Input: part model. Units: mm. Frame: model coordinates. A direction names the side the tool comes from. Give positions to 0.01 mm unless a question says otherwise; leave off trailing zeros. Write each loop counter-clockwise with the first axis right and the second up, starting at its lowest first coordinate (ties: lowest second). Pieces come first, ordered by that corner, then holes. Notation, with made-up numbers: (17, 85) -> (28, 85) arc R11 ccw to (28, 92) -> close; hole circle Ø8 at (47, 79). An arc over 180 degrees is marked (long way). Return JSON: item names as keys, results as strings. Group by question number.
Item 1: Section B-B, the plane z = 22. Return loops of the section in (x, y).
Item 2: Pin query (flat end, axial travel): P1, Ø6.5, axis at x = 10.5, y = -16, coming from the +Z side (3 decimals); P2, Ø1, axis at x = 12, y = -6.5, coming from the +Z side; P3, Ø5.5, axis at x = -20.32, y = -20.32, coming from the +Z side; P4, Ø6.5, axis at x = -20.32, y = 20.32, coming from the -Z side. Return the tip coordinate at first contact, or that it passes through.
Item 3: Section C-C, the plane x = 20.32. Return loops of the section in (y, z) (3 decimals), then the cut area to 3 significant figures.
Item 4: Line query: line 1 (Y direction, x = 20.32, z = 1); line 2 (Z direction, x = 13, y = -16.5) (3 decimals). Output: solid intervals per line, ascending. Write a range as [from, to].
Item 5: Section A-A, the plane y = 20.32. Return loops of the section in (x, z) (3 decimals), then the cut area to 3 significant figures.
Item 6: Set-up query: faces 5 (the face through (-25.4, 0, 2)), 6 (the face through (0, -19, 3.175)), 7 (the face through (0, 19, 3.175)). Return all of +Z, -Z, +X, -X, +Y, -Y with unobstructed straight access to the full face (end or side cutting, diameter ignored); none if empty.
Item 7: Section D-D, the plane y = 10.5. Return loops of the section in (x, z) (3 decimals).
Item 8: Mould query, pull axis X, two halves, no side actions, for faces 1 (the face through (17.879, -0.178, 13.234)), 2 (the face through (-19.228, -22.033, 1.19)), 3 (the face through (0, -12.7, 7)), 4 (the face through (18.82, 18.95, 1.19)). Classes: released by +X, released by -X, zero draft, split by the parting line, or undercut.
from build123d import *

# Parameters (mm, degrees)
F0_W        = 50.8
F0_H        = 50.8
F1_DEPTH    = 3.175
F3_DEPTH    = 12.7
F4_T1_DEPTH = 29.6642315955
F5_R        = 2.032
F6_DEPTH    = 25.4
F7_SIZE     = 0.762


# Not quite as in the source:
# - a fillet or chamfer that OpenCascade refuses, or shapes differently, is made with other operations: its cross-section is extruded or revolved along the edge and cut away or added


with BuildPart() as f1:
    # F0 (on Top) → F1 (new body)
    with BuildSketch(Plane.XY):
        Rectangle(F0_W, F0_H)
    extrude(amount=F1_DEPTH)

    # F2 (on Front) → F3 (join, symmetric)
    with BuildSketch(Plane.XZ):
        with BuildLine():
            ThreePointArc((9.6386223082, 24.257), (0, 9.017), (-9.6386223082, 24.257))
            Line((-9.6386223082, 24.257), (-25.4, 3.175))
            Line((-25.4, 3.175), (25.4, 3.175))
            Line((25.4, 3.175), (9.6386223082, 24.257))
        make_face()
    extrude(amount=F3_DEPTH, both=True)

    # F4: chamfer of 1.016 on 2 edges, made by hand

    # F4_s2 → F4_t1 (cut)
    with BuildSketch(Plane.XZ.offset(-14.8321157977)):
        with BuildLine():
            Line((-10.1809562751, 23.5988049587), (-9.9336646357, 23.4627576649))
            Line((-9.9336646357, 23.4627576649), (-9.9146755466, 23.4555246232))
            ThreePointArc((-9.9146755466, 23.4555246232), (-9.7936995215, 23.8631023282), (-9.6202630276, 24.2482914286))
            Line((-9.6202630276, 24.2482914286), (-9.6548968618, 24.2691672226))
            ThreePointArc((-9.6548968618, 24.2691672226), (-9.9099463042, 23.9280198655), (-10.1972308287, 23.6109721813))
            Line((-10.1972308287, 23.6109721813), (-10.1809562751, 23.5988049587))
        make_face()
        with BuildLine():
            Line((10.1809562751, 23.5988049587), (9.9336646357, 23.4627576649))
            Line((9.9336646357, 23.4627576649), (9.9146755466, 23.4555246232))
            ThreePointArc((9.9146755466, 23.4555246232), (9.7936995215, 23.8631023282), (9.6202630276, 24.2482914286))
            Line((9.6202630276, 24.2482914286), (9.6548968618, 24.2691672226))
            ThreePointArc((9.6548968618, 24.2691672226), (9.9099463042, 23.9280198655), (10.1972308287, 23.6109721813))
            Line((10.1972308287, 23.6109721813), (10.1809562751, 23.5988049587))
        make_face()
    extrude(amount=F4_T1_DEPTH, mode=Mode.SUBTRACT)

    # F5 (on face) → F6 (cut)
    with BuildSketch(Plane(origin=(0, 0, 0), x_dir=(1, 0, 0), z_dir=(0, 0, -1))):
        with Locations((-20.32, 20.32)):
            Circle(F5_R)
        with Locations((-20.32, -20.32)):
            Circle(F5_R)
        with Locations((20.32, 20.32)):
            Circle(F5_R)
        with Locations((20.32, -20.32)):
            Circle(F5_R)
    extrude(amount=-F6_DEPTH, mode=Mode.SUBTRACT)

    # F7
    f7_edges = [f1.edges().sort_by_distance(p)[0] for p in [
        (-22.352, -20.32, 3.175),
        (-22.352, 20.32, 3.175),
        (18.288, 20.32, 3.175),
        (18.288, -20.32, 3.175),
    ]]
    chamfer(f7_edges, length=F7_SIZE)


solid = f1.part
Answer below:
{
 "1": {"outline": "(-11.33, -12.7) -> (-10.41, -12.7) -> (-10.41, 12.7) -> (-11.33, 12.7) -> close; (10.41, -12.7) -> (11.33, -12.7) -> (11.33, 12.7) -> (10.41, 12.7) -> close"},
 "2": {"P1": "stops at z = 3.175", "P2": "stops at z = 21.77", "P3": "stops at z = 3.13", "P4": "stops at z = 0"},
 "3": {"outline": "(-25.4, 0) -> (-22.352, 0) -> (-22.352, 2.413) -> (-23.114, 3.175) -> (-25.4, 3.175) -> close; (-18.288, 0) -> (18.288, 0) -> (18.288, 2.413) -> (17.526, 3.175) -> (12.7, 3.175) -> (12.7, 9.97) -> (-12.7, 9.97) -> (-12.7, 3.175) -> (-17.526, 3.175) -> (-18.288, 2.413) -> close; (22.352, 0) -> (25.4, 0) -> (25.4, 3.175) -> (23.114, 3.175) -> (22.352, 2.413) -> close", "area": "307 mm2"},
 "4": {"line 1": "y = [-25.4, -22.35], [-18.29, 18.29], [22.35, 25.4]", "line 2": "z = [0, 3.175]"},
 "5": {"outline": "(-25.4, 0) -> (-22.352, 0) -> (-22.352, 2.413) -> (-23.114, 3.175) -> (-25.4, 3.175) -> close; (-18.288, 0) -> (18.288, 0) -> (18.288, 2.413) -> (17.526, 3.175) -> (-17.526, 3.175) -> (-18.288, 2.413) -> close; (22.352, 0) -> (25.4, 0) -> (25.4, 3.175) -> (23.114, 3.175) -> (22.352, 2.413) -> close", "area": "134 mm2"},
 "6": {"face 5": "+Z, -Z, -X, +Y, -Y", "face 6": "+Z, +X, -X, -Y", "face 7": "+Z, +X, -X, +Y"},
 "7": {"outline": "(-25.4, 0) -> (25.4, 0) -> (25.4, 3.175) -> (10.145, 23.579) -> (9.969, 23.482) arc R10.668 cw (long way) to (-9.969, 23.482) -> (-10.145, 23.579) -> (-25.4, 3.175) -> close"},
 "8": {"face 1": "released by +X", "face 2": "undercut", "face 3": "zero draft", "face 4": "undercut"}
}
